Source: CAD feature listing. Evaluate the final solid. Frame: model axes, mm. Coordinates: 2 decimals unless noted, no trailing zeros. Order: outer loops, then holes, each group sorted by start corner. A loop starts at its lowest first (then second) coordinate and runs counter-clockwise, first axis right, second up. Notation, with made-up numbers: (-7, -27) -> (4, -27) arc R26 cw to (4, 5) -> close; hole circle Ø2 at (62, 11.5). An arc over 180 degrees is marked (long way). Write each question's results on one line, items separated by ' | '. Start each with the question number.
Autodesk Inventor part; units mm, degrees
ref_plane "YZ Plane" through (0, 0, 0) normal (1, 0, 0) x (0, 1, 0)
ref_plane "XZ Plane" through (0, 0, 0) normal (0, 1, 0) x (-1, 0, 0)
ref_plane "XY Plane" through (0, 0, 0) normal (0, 0, 1) x (1, 0, 0)
sketch "Sketch1" plane through (0, 0, 0) normal (0, 1, 0) x (-1, 0, 0)
  circle A0 centre (0, 0) radius 1
  dimension "d0" = 2
extrude "Extrusion1" add sketch "Sketch1" along normal blind 28
fillet "Fillet1" radius 1 1 edges at (1, 28, 0)
fillet "Fillet2" radius 1 1 edges at (1, 0, 0)
properties part number "pin_2_x_28_mm"
(1) Line query: L1, parallel to Z at x = -0.05, y = 21; L2, parallel to X at y = 10.25, z = 0.1; L3, parallel to Y at x = 0, z = -0.1. Output: solid intervals per line, ascending.
(2) Section A-A on z = 0. Return the cut outline in (x, y).
(3) Section C-C on y = 17. Return the cut outline in (x, z), then the cut area to 3 significant figures.
(4) Section B-B on x = 0. Return the cut outline in (y, z).
Results list:
1) L1: z = -1 to 1 | L2: x = -0.99 to 0.99 | L3: y = 0.01 to 27.99
2) outline: (-1, 1) arc R1 ccw to (1, 1) -> (1, 27) arc R1 ccw to (-1, 27) -> close
3) outline: circle Ø2 at (0, 0) | area: 3.14 mm²
4) outline: (1, -1) -> (27, -1) arc R1 ccw to (27, 1) -> (1, 1) arc R1 ccw to start
